CAD build for the part. Positions are in the model's coordinates, mm. A direction names the side the tool comes from. Coordinates: 2 decimals unless noted, no trailing zeros. Loops run counter-clockwise (first coordinate to the right, second up) from the corner with the lowest first, then second, coordinate; pieces in that order, holes last. Notation, with made-up numbers: (66, 69) - (74, 69) arc R6 cw to (74, 79) - close; hole circle Ø1 at (49, 79.5). An arc over 180 degrees is marked (long way). Put each result on its own line as item: value.
Autodesk Inventor part; units mm, degrees
ref_plane "YZ Plane" through (0, 0, 0) normal (1, 0, 0) x (0, 1, 0)
ref_plane "XZ Plane" through (0, 0, 0) normal (0, 1, 0) x (-1, 0, 0)
ref_plane "XY Plane" through (0, 0, 0) normal (0, 0, 1) x (1, 0, 0)
sketch "Sketch1" plane through (0, 0, 0) normal (0, 0, 1) x (1, 0, 0)
  line L0 (-65.7184, 0) -> (65.7184, 0)
  line L1 (-36.2446, 59.05) -> (36.2446, 59.05)
  circle A0 centre (-30.5, 47) radius 8.55
  line L2 (0, 59.05) -> (0, 0) construction
  circle A1 centre (-30.5, 47) radius 5
  circle A2 centre (30.5, 47) radius 5
  arc A3 (-69.1825, 6) -> (-65.7184, 0) centre (-65.7184, 4) ccw
  arc A4 (-36.2446, 59.05) -> (-39.7087, 57.05) centre (-36.2446, 55.05) ccw
  line L3 (-69.1825, 6) -> (-39.7087, 57.05)
  arc A5 (65.7184, 0) -> (69.1825, 6) centre (65.7184, 4) ccw
  arc A6 (39.7087, 57.05) -> (36.2446, 59.05) centre (36.2446, 55.05) ccw
  line L4 (69.1825, 6) -> (39.7087, 57.05)
  line L5 (-65.7184, 3) -> (-30.5, 3)
  line L6 (-30.5, 3) -> (-30.5, 0)
  line L7 (-30.5, 0) -> (-65.7184, 0)
  line L8 (-65.7184, 0) -> (-65.7184, 3)
  line L9 (-30.5, 38.45) -> (0, 38.45) construction
  line L10 (-30.5, 3) -> (0, 3) construction
  line L11 (0, 38.45) -> (0, 3) construction
  line L12 (-60.5222, 9) -> (-47.5607, 31.45)
  line L13 (-47.5607, 31.45) -> (47.5607, 31.45)
  line L14 (47.5607, 31.45) -> (60.5222, 9)
  line L15 (60.5222, 9) -> (-60.5222, 9)
  circle A7 centre (30.5, 47) radius 9.55
  point P0 (-65.7184, 1.5)
  point P1 (-48.1092, 0)
  point P2 (-65.7184, 0)
  point P3 (-30.5, 0)
  point P4 (-30.5, 1.5)
  point P5 (0, 20.725)
  point P6 (0, 20.725)
  point P7 (0, 20.725)
  dimension "d1" = 17.1
  dimension "d3" = 3.5
  dimension "d7" = 10
  dimension "d10" = 4
  dimension "d11" = 13
  dimension "d12" = 60
  dimension "d17" = 3
  dimension "d22" = 44
  dimension "d40" = 6
  dimension "d41" = 6
  dimension "d43" = 6
  dimension "d44" = 19.1
  dimension "d45" = 61
  dimension "d46" = 6
extrude "Extrusion1" add sketch "Sketch1" along normal mid plane 30 contours A3 L3 A4 L1 A6 L4 A5 L0 L6 L5 L8
extrude "Extrusion2" add sketch "Sketch1" along normal mid plane 20 contours A0 | A7
extrude "Extrusion3" add sketch "Sketch1" along normal blind 27.5 contours L8 L5 L6 L0
sketch "Sketch2" plane through (-65.7184, 3, 15) normal (0, 1, 0) x (1, 0, 0)
  line L0 (0, -12.5) -> (35.2184, -12.5)
  arc A0 (20.1092, -12.5) -> (15.1092, -12.5) centre (17.6092, -8.1699) ccw
  line L1 (35.2184, 0) -> (131.4367, 0) construction
  line L2 (35.2184, 0) -> (35.2184, -12.5) construction
  point P0 (65.7184, 15)
  point P1 (17.6092, -12.5)
  point P2 (17.6092, -3.1699)
  dimension "d21" = 5
  dimension "d25" = 5
extrude "Extrusion4" cut sketch "Sketch2" against normal through all
extrude "Extrusion6" add sketch "Sketch1" against normal blind 15 contours L8 L5 L6 L0
properties part number "EngineMount - Big hole"
Q1. Mould opens along X. For faces 1 (the flat face through (-1, 0, 2)), 2 (the cylindrical face through (28.43, 56.323, 12.465)), 3 (the cylindrical face through (-69.153, 1.949, -0.21)) say: +X half, -X half, draft (parallel to the pull), parting line (faces both ways), or undercut.
Determined:
face 1: draft
face 2: undercut
face 3: -X half
Q2. Slice it at D-D, the plane z = 24. Give the cut face in (x, y), then the cut area to 3 significant figures.
Determined:
outline: (-65.72, 0) - (-53.04, 0) - (-53.04, 3) - (-65.72, 3) - close; (-43.18, 0) - (-30.5, 0) - (-30.5, 3) - (-43.18, 3) - close
area: 76.1 mm2
Q3. Slice it at A-A, the plane z = 11.5. Give the cut face in (x, y), then the cut area to 3 significant figures.
Determined:
outline: (-69.18, 6) arc R4 ccw to (-65.72, 0) - (65.72, 0) arc R4 ccw to (69.18, 6) - (39.71, 57.05) arc R4 ccw to (36.24, 59.05) - (-36.24, 59.05) arc R4 ccw to (-39.71, 57.05) - close; hole (-60.52, 9) - (60.52, 9) - (47.56, 31.45) - (-47.56, 31.45) - close; hole circle Ø17.1 at (-30.5, 47); hole circle Ø19.1 at (30.5, 47)
area: 3,600 mm2
Q4. Pin check, flat tips, straight feed: pin 1 Ø13.5 at (x, y) = (-27, 45.5) entering from -Z; pin 2 Ø21 at (x, y) = (35, 49.5) entering from +Z; pin 3 Ø3.5 at (y, z) = (1, 23) entering from -X; pin 4 Ø15.5 at (x, y) = (30.5, 47) entering from +Z. Stop position of each tip, or through.
Determined:
pin 1: z = -15
pin 2: z = 15
pin 3: x = -65.72
pin 4: z = 10
Q5. Tool access for faces 4 (the flat face through (-27, 43, 10)), 5 (the flat face through (-30.5, 2, 21)), 6 (the cylindrical face through (28.43, 56.323, -12.535)), 7 (the cylindrical face through (-38.27, 58.5, -0.21)), 8 (the flat face through (-1, 31.45, 0)): list every direction of +Z, -Z, +X, -X, +Y, -Y with a clear straight run to the whole face (end or side of a thin tool).
Determined:
face 4: +Z
face 5: +Z, +X, +Y, -Y
face 6: -Z
face 7: +Z, -Z, -X, +Y
face 8: +Z, -Z
Q6. Slice it at C-C, the plane x = 30.5. Give the cut face in (y, z), then the cut area to 3 significant figures.
Determined:
outline: (0, -15) - (9, -15) - (9, 15) - (0, 15) - close; (31.45, -15) - (37.45, -15) - (37.45, -10) - (42, -10) - (42, 10) - (37.45, 10) - (37.45, 15) - (31.45, 15) - close; (52, -10) - (56.55, -10) - (56.55, -15) - (59.05, -15) - (59.05, 15) - (56.55, 15) - (56.55, 10) - (52, 10) - close
area: 707 mm2
Q7. Slice it at B-B, the plane y = 47. Give the cut face in (x, z), then the cut area to 3 significant figures.
Determined:
outline: (-45.51, -15) - (-39.05, -15) - (-39.05, -10) - (-35.5, -10) - (-35.5, 10) - (-39.05, 10) - (-39.05, 15) - (-45.51, 15) - close; (-25.5, -10) - (-21.95, -10) - (-21.95, -15) - (20.95, -15) - (20.95, -10) - (25.5, -10) - (25.5, 10) - (20.95, 10) - (20.95, 15) - (-21.95, 15) - (-21.95, 10) - (-25.5, 10) - close; (35.5, -10) - (40.05, -10) - (40.05, -15) - (45.51, -15) - (45.51, 15) - (40.05, 15) - (40.05, 10) - (35.5, 10) - close
area: 1,970 mm2
Q8. Wall check: L1, parallel to Y at x = 30.5, z = -11.6; L2, parallel to Y at x = -30.5, z = 13; L3, parallel to Y at x = -6.5, z = 1.5. Give the ranges that are in metal, low to high. Write a range as from..to.
Determined:
L1: 0..9, 31.45..37.45, 56.55..59.05
L2: 0..9, 31.45..38.45, 55.55..59.05
L3: 0..9, 31.45..59.05
